Geometry: final body of the model. Coordinates: model frame, mm. A direction names the side the tool comes from. Give positions to 0.01 mm unless a question says otherwise; leave off trailing zeros. Loops run counter-clockwise (first coordinate to the right, second up) from the corner with the lowest first, then second, coordinate; pieces in that order, holes last. Notation, with made-up numbers: (-11.5, 26.25) -> (39.5, 26.25) arc R30 cw to (39.5, 65.25) -> close; hole circle Ø6 at (-18, 80). An arc over 180 degrees is marked (long way). Answer in a Markdown table with one row per item. Add a question column.
1) Section query B-B (z = 29). Return the cut outline in (x, y) (3 decimals), plus the area to 3 significant figures.
2) First-contact query: P1, Ø1.8, axis at x = -2, y = 0.5, coming from the -Z side; P2, Ø0.7, axis at y = -1, z = 25, coming from the -X side (3 decimals); P3, Ø1.8, axis at x = -2.5, y = 0, coming from the +Z side. Flat tips, straight axial feed; report the tip coordinate or a pass-through.
3) Access query for faces 4 (the flat face through (8, 0, -6)), 5 (the flat face through (26, 0, 17.9)), 6 (the flat face through (-3.58, 0, 18.8)), 7 (the cylindrical face through (20.99, 0.41, 8.21)), 8 (the cylindrical face through (-5.34, 0.06, 8.15)). Directions: +Z, -Z, +X, -X, +Y, -Y. A direction counts if a zero-diameter tool reaches every point of the face in a straight line with its end or side. Return the directions, or none.
4) Draft query along X for faces 1 (the flat face through (2, 0, 24.125)), 2 (the flat face through (8, 0, 35.8)), 3 (the flat face through (22.745, 0, 24)). Return one class per face: +X half, -X half, draft (parallel to the pull), parting line (faces both ways), or undercut.
5) Section query D-D (x = -6). Return the cut outline in (y, z).
6) Line query: line 1 (X direction, y = -1.5, z = 7.5) (3 decimals); line 2 (Z direction, x = 15, y = -0.9) (3 decimals); line 3 (X direction, y = 1.45, z = 25) (3 decimals). Output: solid intervals per line, ascending. Write a range as from..to.
7) Section query C-C (y = 2). Give the number of separate pieces and of enclosed holes in the cut face, plus the area to 3 significant figures.
8) Section query A-A (x = 0.5). Return the cut outline in (y, z) (3 decimals).
Autodesk Inventor part; units mm, degrees
ref_plane "작업 평면4" through (10.8037, 3, 0) normal (0, 1, 0) x (1, 0, 0)
ref_plane "YZ Plane" through (0, 0, 0) normal (1, 0, 0) x (0, 1, 0)
ref_plane "XZ Plane" through (0, 0, 0) normal (0, 1, 0) x (-1, 0, 0)
sketch "스케치1" plane through (0, 0, 0) normal (0, 0, 1) x (1, 0, 0)
  arc A0 (-4.555, 20.4) -> (-1.5118, 17.2038) centre (-1.355, 20.4) ccw
  line L0 (-4.555, 20.4) -> (-4.555, 29.4)
  line L1 (-4.555, 29.4) -> (-9.955, 29.4)
  line L2 (-9.955, 29.4) -> (-9.955, 17.8)
  line L3 (-9.955, 17.8) -> (-4.855, 11.8)
  line L4 (-4.855, 11.8) -> (-4.7625, 11.8)
  line L5 (-4.7625, 11.8) -> (-4.7625, -3)
  line L6 (-4.7625, -3) -> (3.7037, -3)
  arc A1 (4.7037, -2) -> (3.7037, -3) centre (4.7037, -3) ccw
  line L7 (4.7037, -2) -> (4.7037, 2.1)
  arc A2 (5.6987, 3) -> (4.7037, 2.1) centre (4.7037, 3.1) ccw
  line L8 (5.6987, 3) -> (9.9088, 3)
  arc A3 (10.9037, 2.1) -> (9.9088, 3) centre (10.9037, 3.1) ccw
  line L9 (10.9037, 2.1) -> (10.9037, -2)
  arc A4 (11.9037, -3) -> (10.9037, -2) centre (10.9037, -3) ccw
  line L10 (11.9037, -3) -> (20.4525, -3)
  line L11 (20.4525, -3) -> (20.4525, 11.8)
  line L12 (20.4525, 11.8) -> (20.545, 11.8)
  line L13 (20.545, 11.8) -> (25.645, 17.8)
  line L14 (25.645, 17.8) -> (25.645, 29.4)
  line L15 (25.645, 29.4) -> (20.245, 29.4)
  line L16 (20.245, 29.4) -> (20.245, 20.4)
  arc A5 (17.2018, 17.2038) -> (20.245, 20.4) centre (17.045, 20.4) ccw
  line L17 (17.2018, 17.2038) -> (-1.5118, 17.2038)
  circle A6 centre (13.2469, 0) radius 1.35
  circle A7 centre (2.4432, 0) radius 1.35
  circle A8 centre (18.0506, 0) radius 1.35
  circle A9 centre (-2.3606, 0) radius 1.35
  circle A10 centre (-7.155, 20.9) radius 1.35
  circle A11 centre (-0.655, 14.6) radius 1.35
  circle A12 centre (16.345, 14.6) radius 1.35
  circle A13 centre (22.845, 20.9) radius 1.35
  line L18 (20.4525, -3) -> (-4.855, -3)
  line L19 (-4.855, -3) -> (-4.855, 3)
  line L20 (-4.855, 3) -> (20.4525, 3)
  line L21 (20.4525, 3) -> (20.4525, -3)
  line L22 (22.845, 3) -> (22.845, -11.8)
  line L23 (-7.155, 3) -> (-7.155, -11.8)
  line L24 (22.745, 3) -> (22.745, -11.8)
  line L25 (-7.055, 3) -> (-7.055, -11.8)
  line L26 (22.745, -3) -> (-7.055, -3)
  line L27 (-7.055, -3) -> (-7.055, 3)
  line L28 (-7.055, 3) -> (22.745, 3)
  line L29 (22.745, 3) -> (22.745, -3)
  point P0 (0, 0)
  point P1 (11.8625, -3)
  point P2 (20.4525, 3)
  point P3 (9.8675, 3)
  point P4 (5.6574, 3)
  point P5 (-4.7625, 3)
  point P6 (3.6625, -3)
  point P7 (-4.855, 3)
  point P8 (-7.055, -3)
  point P9 (-4.855, -3)
  point P10 (-4.7625, -3)
  point P11 (22.745, 1.2049)
  point P12 (20.4525, 3)
  point P13 (20.4525, -3)
  point P14 (11.8987, 3)
  point P15 (3.7037, -3)
  point P16 (11.9037, -3)
  point P17 (5.6987, 3)
  point P18 (3.7088, 3)
  point P19 (5.6987, 3)
  point P20 (11.9037, -3)
  point P21 (-4.7625, 3)
  point P22 (-4.855, -3)
  point P23 (10.9037, -1.792)
  point P24 (-4.7625, -3)
  point P25 (4.7037, -1.792)
  dimension "d7" = 0.1
  dimension "d8" = 0.1
extrude "돌출1" add sketch "스케치1" along normal blind 29.8 contours L20 A2 L7 A1 L6 L5 | L5 L18 L19 L20 | L19 L26 L25 L28 | L20 L8 A3 L9 A4 L18 A1 L7 A2 | L28 L24 L26 L11 | L11 L10 A4 L9 A3 L20 | A6 | A7 | A8 | A9
ref_plane "작업 평면4" through (10.8037, 3, 0) normal (0, 1, 0) x (1, 0, 0)
sketch "스케치5" plane through (10.8037, 3, 0) normal (0, 1, 0) x (1, 0, 0)
  line L0 (1.1931, -3.675) -> (1.1931, 6)
  line L1 (3.6931, -3.675) -> (3.6931, 6)
  line L2 (1.1931, -5.675) -> (3.6931, -5.675)
  line L3 (2.4431, 0) -> (2.4431, -3.675)
  line L4 (2.4431, -5.675) -> (2.4431, -4.575)
  line L5 (2.4431, -4.575) -> (2.4431, -3.475)
  line L6 (2.4431, -3.475) -> (-0.1069, -3.475)
  line L7 (2.4431, -3.475) -> (4.9931, -3.475)
  line L8 (4.9931, -3.475) -> (-0.1069, -3.475)
  line L9 (-0.1069, -3.475) -> (-0.1069, -5.675)
  line L10 (-0.1069, -5.675) -> (4.9931, -5.675)
  line L11 (4.9931, -5.675) -> (4.9931, -3.475)
  line L12 (1.1931, -5.675) -> (1.1931, 6)
  line L13 (3.6931, -5.675) -> (3.6931, 6)
  line L14 (1.1931, -5.675) -> (3.6931, -5.675)
  line L15 (2.4431, -3.675) -> (2.4431, -5.675)
  line L16 (-23.9, -14.9) -> (17.9, -14.9)
  line L17 (1.1931, -24.125) -> (3.6931, -24.125)
  line L18 (2.4431, -24.125) -> (2.4431, -25.225)
  line L19 (2.4431, -25.225) -> (2.4431, -26.325)
  line L20 (2.4431, -26.325) -> (-0.1069, -26.325)
  line L21 (2.4431, -26.325) -> (4.9931, -26.325)
  line L22 (4.9931, -26.325) -> (-0.1069, -26.325)
  line L23 (-0.1069, -26.325) -> (-0.1069, -24.125)
  line L24 (-0.1069, -24.125) -> (4.9931, -24.125)
  line L25 (4.9931, -24.125) -> (4.9931, -26.325)
  line L26 (1.1931, -24.125) -> (3.6931, -24.125)
  line L27 (2.4431, -26.125) -> (2.4431, -24.125)
  line L28 (-3, -14.9) -> (-3, -22)
  line L29 (-7.1931, -5.675) -> (-9.6931, -5.675)
  line L30 (-8.4431, -5.675) -> (-8.4431, -4.575)
  line L31 (-8.4431, -4.575) -> (-8.4431, -3.475)
  line L32 (-8.4431, -3.475) -> (-5.8931, -3.475)
  line L33 (-8.4431, -3.475) -> (-10.9931, -3.475)
  line L34 (-10.9931, -3.475) -> (-5.8931, -3.475)
  line L35 (-5.8931, -3.475) -> (-5.8931, -5.675)
  line L36 (-5.8931, -5.675) -> (-10.9931, -5.675)
  line L37 (-10.9931, -5.675) -> (-10.9931, -3.475)
  line L38 (-7.1931, -5.675) -> (-9.6931, -5.675)
  line L39 (-8.4431, -3.675) -> (-8.4431, -5.675)
  line L40 (-7.1931, -24.125) -> (-9.6931, -24.125)
  line L41 (-8.4431, -24.125) -> (-8.4431, -25.225)
  line L42 (-8.4431, -25.225) -> (-8.4431, -26.325)
  line L43 (-7.1931, -24.125) -> (-9.6931, -24.125)
  line L44 (-8.4431, -26.125) -> (-8.4431, -24.125)
  line L45 (-8.4431, -26.325) -> (-10.9931, -26.325)
  line L46 (-10.9931, -24.125) -> (-10.9931, -26.325)
  line L47 (-8.4431, -26.325) -> (-5.8931, -26.325)
  line L48 (-5.8931, -26.325) -> (-5.8931, -24.125)
  line L49 (-10.9931, -26.325) -> (-5.8931, -26.325)
  line L50 (-5.8931, -24.125) -> (-10.9931, -24.125)
  line L51 (-12.1837, -21.5519) -> (-23.8587, -21.5519)
  line L52 (-12.1837, -19.0519) -> (-23.8587, -19.0519)
  line L53 (-12.1837, -19.0519) -> (-12.1837, -21.5519)
  line L54 (-12.1837, -19.0519) -> (-14.3837, -19.0519)
  line L55 (-12.1837, -20.3019) -> (-12.1837, -18.0519)
  line L56 (-12.1837, -20.3019) -> (-12.1837, -22.5519)
  line L57 (-14.3837, -18.0519) -> (-12.1837, -18.0519)
  line L58 (-12.1837, -18.0519) -> (-12.1837, -22.5519)
  line L59 (-12.1837, -22.5519) -> (-14.3837, -22.5519)
  line L60 (-14.3837, -22.5519) -> (-14.3837, -18.0519)
  line L61 (-12.1837, -10.7481) -> (-12.1837, -8.2481)
  line L62 (-12.1837, -10.7481) -> (-14.3837, -10.7481)
  line L63 (-12.1837, -9.4981) -> (-12.1837, -11.7481)
  line L64 (-12.1837, -9.4981) -> (-12.1837, -7.2481)
  line L65 (-14.3837, -11.7481) -> (-12.1837, -11.7481)
  line L66 (-12.1837, -11.7481) -> (-12.1837, -7.2481)
  line L67 (-12.1837, -7.2481) -> (-14.3837, -7.2481)
  line L68 (-14.3837, -7.2481) -> (-14.3837, -11.7481)
  line L69 (6.1837, -19.0519) -> (6.1837, -21.5519)
  line L70 (6.1837, -19.0519) -> (8.3837, -19.0519)
  line L71 (6.1837, -20.3019) -> (6.1837, -18.0519)
  line L72 (6.1837, -20.3019) -> (6.1837, -22.5519)
  line L73 (8.3837, -18.0519) -> (6.1837, -18.0519)
  line L74 (6.1837, -18.0519) -> (6.1837, -22.5519)
  line L75 (6.1837, -22.5519) -> (8.3837, -22.5519)
  line L76 (8.3837, -22.5519) -> (8.3837, -18.0519)
  line L77 (6.1837, -9.4981) -> (6.1837, -7.2481)
  line L78 (6.1837, -7.2481) -> (8.3837, -7.2481)
  line L79 (6.1837, -10.7481) -> (6.1837, -8.2481)
  line L80 (6.1837, -9.4981) -> (6.1837, -11.7481)
  line L81 (6.1837, -10.7481) -> (8.3837, -10.7481)
  line L82 (8.3837, -11.7481) -> (6.1837, -11.7481)
  line L83 (8.3837, -7.2481) -> (8.3837, -11.7481)
  line L84 (6.1837, -11.7481) -> (6.1837, -7.2481)
  point P0 (-0.1069, -3.475)
  point P1 (1.1931, -26.125)
  point P2 (3.6931, -26.125)
  point P3 (-7.1931, -3.675)
  point P4 (-9.6931, -3.675)
  point P5 (-7.1931, -26.125)
  point P6 (-9.6931, -26.125)
  point P7 (-0.1069, -26.325)
  point P8 (3.6931, -24.125)
  point P9 (1.1931, -24.125)
  dimension "d24" = 1.1
  dimension "d25" = 1.1
  dimension "d26" = 2.55
  dimension "d27" = 2.55
  dimension "d28" = 2.2
  dimension "d29" = 2.25
  dimension "d30" = 2.25
extrude "돌출4" cut sketch "스케치5" against normal blind 6
sketch "스케치6" plane through (-7.055, -3, 29.8) normal (-1, 0, 0) x (0, 0, 1)
  circle A0 centre (-9.4981, 3) radius 1.35
  circle A1 centre (-20.3019, 3) radius 1.35
  point P0 (-29.8, 3)
extrude "돌출5" cut sketch "스케치6" against normal up to next
sketch "스케치7" plane through (0, 0, 0) normal (0, 0, -1) x (-1, 0, 0)
  circle A0 centre (-13.2469, 0) radius 1.35
  circle A1 centre (-2.4432, 0) radius 1.35
  point P0 (0, 0)
extrude "돌출6" cut sketch "스케치7" against normal up to next
sketch "스케치8" plane through (22.745, -3, 0) normal (1, 0, 0) x (0, 0, -1)
  circle A0 centre (-20.3019, 3) radius 1.35
  circle A1 centre (-9.4981, 3) radius 1.35
  point P0 (0, 3)
extrude "돌출7" cut sketch "스케치8" against normal up to next
sketch "스케치9" plane through (0, 0, 29.8) normal (0, 0, 1) x (1, 0, 0)
  circle A0 centre (2.4432, 0) radius 1.35
  circle A1 centre (13.2469, 0) radius 1.35
  point P0 (0, 0)
extrude "돌출8" cut sketch "스케치9" against normal up to next
sketch "스케치10" plane through (-7.055, 3, 0) normal (0, 1, 0) x (1, 0, 0)
  line L0 (24.0424, -18.0519) -> (26.2424, -18.0519)
  line L1 (26.2424, -18.0519) -> (26.2424, -22.5519)
  line L2 (26.2424, -22.5519) -> (24.0424, -22.5519)
  line L3 (24.0424, -22.5519) -> (24.0424, -18.0519)
  line L4 (11.9656, -3.475) -> (11.9656, -5.675)
  line L5 (11.9656, -5.675) -> (6.8656, -5.675)
  line L6 (6.8656, -5.675) -> (6.8656, -3.475)
  line L7 (6.8656, -3.475) -> (11.9656, -3.475)
  line L8 (11.9656, -24.125) -> (11.9656, -26.325)
  line L9 (11.9656, -26.325) -> (6.8656, -26.325)
  line L10 (6.8656, -26.325) -> (6.8656, -24.125)
  line L11 (6.8656, -24.125) -> (11.9656, -24.125)
  line L12 (3.475, -7.2481) -> (5.675, -7.2481)
  line L13 (5.675, -7.2481) -> (5.675, -11.7481)
  line L14 (5.675, -11.7481) -> (3.475, -11.7481)
  line L15 (3.475, -11.7481) -> (3.475, -7.2481)
  line L16 (26.2424, -11.7481) -> (24.0424, -11.7481)
  line L17 (24.0424, -11.7481) -> (24.0424, -7.2481)
  line L18 (24.0424, -7.2481) -> (26.2424, -7.2481)
  line L19 (26.2424, -7.2481) -> (26.2424, -11.7481)
  line L20 (22.8519, -3.475) -> (22.8519, -5.675)
  line L21 (22.8519, -5.675) -> (17.7519, -5.675)
  line L22 (17.7519, -5.675) -> (17.7519, -3.475)
  line L23 (17.7519, -3.475) -> (22.8519, -3.475)
  line L24 (22.8519, -24.125) -> (22.8519, -26.325)
  line L25 (22.8519, -26.325) -> (17.7519, -26.325)
  line L26 (17.7519, -26.325) -> (17.7519, -24.125)
  line L27 (17.7519, -24.125) -> (22.8519, -24.125)
  line L28 (3.475, -18.0519) -> (5.675, -18.0519)
  line L29 (5.675, -18.0519) -> (5.675, -22.5519)
  line L30 (5.675, -22.5519) -> (3.475, -22.5519)
  line L31 (3.475, -22.5519) -> (3.475, -18.0519)
  line L32 (29.8, 0) -> (0, 0)
  line L33 (0, 0) -> (0, -29.8)
  line L34 (29.8, -29.8) -> (0, -29.8)
  line L35 (29.8, 0) -> (29.8, -29.8)
  line L36 (0, -14.9) -> (-6, -14.9)
  line L37 (-6, -14.9) -> (-6, -11.9)
  line L38 (-6, -11.9) -> (0, -11.9)
  line L39 (0, -11.9) -> (0, -17.9)
  line L40 (0, -17.9) -> (-6, -17.9)
  line L41 (-6, -17.9) -> (-6, -11.9)
  line L42 (14.9, 0) -> (14.9, -2)
  line L43 (29.8, -14.9) -> (35.8, -14.9)
  line L44 (35.8, -14.9) -> (35.8, -11.9)
  line L45 (35.8, -11.9) -> (29.8, -11.9)
  line L46 (29.8, -11.9) -> (29.8, -17.9)
  line L47 (29.8, -17.9) -> (35.8, -17.9)
  line L48 (35.8, -17.9) -> (35.8, -11.9)
  line L49 (14.9, 0) -> (14.9, 3)
  line L50 (14.9, 3) -> (14.9, 6)
  line L51 (14.9, 6) -> (11.9, 6)
  line L52 (11.9, 6) -> (17.9, 6)
  line L53 (17.9, 6) -> (17.9, 0)
  line L54 (17.9, 0) -> (11.9, 0)
  line L55 (11.9, 0) -> (11.9, 6)
  line L56 (14.9, -29.8) -> (14.9, -32.8)
  line L57 (14.9, -32.8) -> (14.9, -35.8)
  line L58 (14.9, -35.8) -> (11.9, -35.8)
  line L59 (11.9, -35.8) -> (17.9, -35.8)
  line L60 (17.9, -35.8) -> (17.9, -29.8)
  line L61 (17.9, -29.8) -> (11.9, -29.8)
  line L62 (11.9, -29.8) -> (11.9, -35.8)
  point P0 (7.055, 0)
  point P1 (0, -11.9)
  dimension "d39" = 3
  dimension "d40" = 6
  dimension "d41" = 3
  dimension "d42" = 6
extrude "돌출9" add sketch "스케치10" against normal blind 6 contours L32 L49 L50 L52 L53 | L45 L44 L43 L35 | L32 L55 L51 L50 L49 | L43 L48 L47 L35 | L33 L36 L37 L38 | L60 L59 L57 L56 L34 | L33 L40 L41 L36 | L56 L57 L58 L62 L34
properties part number "arm_motor_connect"
Evaluation:
| question | item | result |
|---|---|---|
| 1 | outline | (-7.055, -3) -> (22.745, -3) -> (22.745, 3) -> (-7.055, 3) -> close; hole circle Ø2.7 at (2.443, 0); hole circle Ø2.7 at (13.247, 0) |
| 1 | area | 167 mm² |
| 2 | P1 | z = 0 |
| 2 | P2 | x = -7.055 |
| 2 | P3 | z = 29.8 |
| 3 | face 4 | -Z, +X, -X, +Y, -Y |
| 3 | face 5 | +Z, +X, +Y, -Y |
| 3 | face 6 | +Y, -Y |
| 3 | face 7 | +X |
| 3 | face 8 | -X |
| 4 | face 1 | undercut |
| 4 | face 2 | draft |
| 4 | face 3 | +X half |
| 5 | outline | (-3, 0) -> (3, 0) -> (3, 29.8) -> (-3, 29.8) -> close; hole circle Ø2.7 at (0, 9.5); hole circle Ø2.7 at (0, 20.3) |
| 6 | line 1 | -7.055..-3.58, -1.38..16.987, 19.187..22.745 |
| 6 | line 2 | 0..3.475, 5.675..24.125, 26.325..29.8 |
| 6 | line 3 | -7.055..-0.189, 4.911..10.697, 15.797..22.745 |
| 7 | separate pieces | 1 |
| 7 | enclosed holes | 8 |
| 7 | area | 948 mm² |
| 8 | outline | (-3, 0) -> (3, 0) -> (3, 3.475) -> (-3, 3.475) -> close; (-3, 5.675) -> (3, 5.675) -> (3, 24.125) -> (-3, 24.125) -> close; (-3, 26.325) -> (3, 26.325) -> (3, 29.8) -> (-3, 29.8) -> close |
